Part model, mm, in its own coordinate system. Face numbers are marked on the shaded views. A direction names the side the tool comes from. Round coordinates to 2 decimals unless told otherwise and drop trailing zeros. Loops run counter-clockwise (first coordinate to the right, second up) from the corner with the lowest first, then second, coordinate; pieces in that order, holes last. Notation, with made-up numbers: (52.25, -9.75) -> (100.25, -9.75) arc R30 ccw to (100.25, 23.25) -> close; hole circle Ø3 at (19.25, 59.5). An arc over 180 degrees is marked (long way). Use a Markdown table: item, result. Add a question column.
Item 1: Cut at C-C, the plane y = 24. List the corners of the cut face in (x, z).
Item 2: Cut at B-B, the plane z = 16. List the corners of the cut face in (x, y).
Item 3: Flat gauge pins, fed straight in: pin 1 (1.6 mm diameter, centred on x = -27.5, z = 7.5, fed in from +Y); pin 2 (3.5 mm diameter, centred on x = -28.5, y = -2.5, fed in from +Z); pin 3 (3.5 mm diameter, centred on x = -28, z = 2.5, fed in from -Y). Where does each tip first touch, or does it go through?
Item 4: Probe line 1 (Y direction, x = 44, z = 6.75); line 2 (X direction, y = 17.5, z = 12.5); line 3 (Y direction, x = -3.5, z = 5.75). List the from-to ranges inside material, lowest first. Write a range as [from, to].
Item 5: Cut at A-A, the plane x = 26. List the corners of the cut face in (y, z), plus the area to 3 significant figures.
Item 6: Which spindle directions (+Z, -Z, +X, -X, +Y, -Y) get a long thin tool onto all of the face, cutting with end or side? Do the marked faces 1 and 2. Say none if no direction does.
Item 7: Cut at D-D, the plane y = 0. List the corners of the cut face in (x, z), plus the area to 3 significant figures.
Item 8: Two-plate mould, pull along X, no slides. Class the marked faces 3, 4, 5 and 6: pulls with the +X half, pulls with the -X half, needs draft (parallel to the pull), parting line crosses it, or undercut.
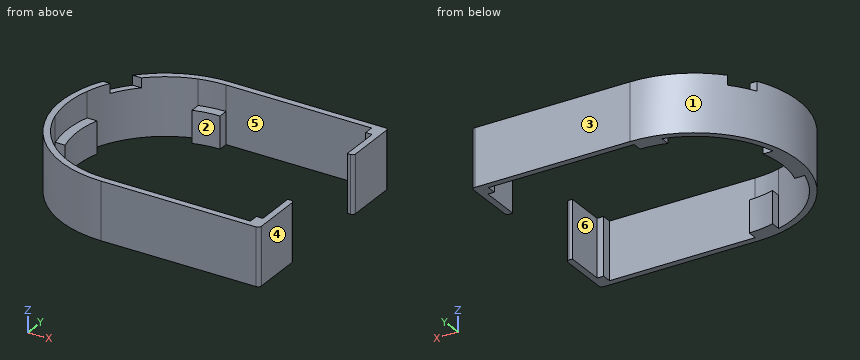
```python
from build123d import *

# Parameters (mm, degrees)
F1_DEPTH = 18
F2_R     = 1
F3_DEPTH = 10
F5_DEPTH = 3


with BuildPart() as f1:
    # F0 (on Top) → F1 (new body)
    with BuildSketch(Plane.XY):
        with BuildLine():
            Line((49.5, -32.5), (49.5, -15))
            Line((49.5, -15), (47.5, -15))
            Line((47.5, -15), (47.5, -27.5))
            Line((47.5, -27.5), (45.5, -27.5))
            Line((45.5, -27.5), (45.5, -30.5))
            Line((45.5, -30.5), (0, -30.5))
            ThreePointArc((0, -30.5), (-4.0354787933, -30.2318525881), (-8, -29.4321253055))
            ThreePointArc((-8, -29.4321253055), (-21.5667568262, -21.5667568262), (-29.4321253055, -8))
            ThreePointArc((-29.4321253055, -8), (-30.5, 0), (-29.4321253055, 8))
            ThreePointArc((-29.4321253055, 8), (-21.5667568262, 21.5667568262), (-8, 29.4321253055))
            ThreePointArc((-8, 29.4321253055), (-4.0354787933, 30.2318525881), (0, 30.5))
            Line((0, 30.5), (45.5, 30.5))
            Line((45.5, 30.5), (45.5, 27.5))
            Line((45.5, 27.5), (47.5, 27.5))
            Line((47.5, 27.5), (47.5, 15))
            Line((47.5, 15), (49.5, 15))
            Line((49.5, 15), (49.5, 32.5))
            Line((49.5, 32.5), (0, 32.5))
            ThreePointArc((0, 32.5), (-32.5, 0), (0, -32.5))
            Line((0, -32.5), (49.5, -32.5))
        make_face()
    extrude(amount=F1_DEPTH)

    # F2
    f2_edges = [f1.edges().sort_by_distance(p)[0] for p in [
        (49.5, 15, 9),
        (49.5, -15, 9),
        (49.5, 32.5, 9),
        (49.5, -32.5, 9),
    ]]
    fillet(f2_edges, radius=F2_R)

    # F0 (on Top) → F3 (join)
    with BuildSketch(Plane.XY):
        with BuildLine():
            ThreePointArc((0, 30.5), (-4.0354787933, 30.2318525881), (-8, 29.4321253055))
            Line((-8, 29.4321253055), (-8, 26.3106442338))
            ThreePointArc((-8, 26.3106442338), (-4.0439636231, 27.2010359769), (0, 27.5))
            Line((0, 27.5), (0, 30.5))
        make_face()
        with BuildLine():
            ThreePointArc((-29.4321253055, 8), (-30.5, 0), (-29.4321253055, -8))
            Line((-29.4321253055, -8), (-26.3106442338, -8))
            ThreePointArc((-26.3106442338, -8), (-27.5, 0), (-26.3106442338, 8))
            Line((-26.3106442338, 8), (-29.4321253055, 8))
        make_face()
        with BuildLine():
            ThreePointArc((-8, -29.4321253055), (-4.0354787933, -30.2318525881), (0, -30.5))
            Line((0, -30.5), (0, -27.5))
            ThreePointArc((0, -27.5), (-4.0439636231, -27.2010359769), (-8, -26.3106442338))
            Line((-8, -26.3106442338), (-8, -29.4321253055))
        make_face()
    extrude(amount=F3_DEPTH)

    # F4 (on face) → F5 (cut)
    with BuildSketch(Plane.XY.offset(18)):
        with BuildLine():
            Line((-28.8314064867, 15), (-26.5565434498, 15))
            ThreePointArc((-26.5565434498, 15), (-24.0961320452, 18.698299935), (-21.1246301743, 22))
            Line((-21.1246301743, 22), (-23.9217474278, 22))
            ThreePointArc((-23.9217474278, 22), (-26.6077772837, 18.6621592539), (-28.8314064867, 15))
        make_face()
    extrude(amount=-F5_DEPTH, mode=Mode.SUBTRACT)


solid = f1.part
```
A:
| question | item | result |
|---|---|---|
| 1 | outline | (-21.91, 0) -> (-18.82, 0) -> (-18.82, 18) -> (-21.91, 18) -> close; (47.5, 0) -> (49.5, 0) -> (49.5, 18) -> (47.5, 18) -> close |
| 2 | outline | (-28.83, 15) arc R32.5 ccw to (0, -32.5) -> (48.5, -32.5) arc R1 ccw to (49.5, -31.5) -> (49.5, -16) arc R1 ccw to (48.5, -15) -> (47.5, -15) -> (47.5, -27.5) -> (45.5, -27.5) -> (45.5, -30.5) -> (0, -30.5) arc R30.5 cw to (-26.56, 15) -> close; (-23.92, 22) -> (-21.12, 22) arc R30.5 cw to (0, 30.5) -> (45.5, 30.5) -> (45.5, 27.5) -> (47.5, 27.5) -> (47.5, 15) -> (48.5, 15) arc R1 ccw to (49.5, 16) -> (49.5, 31.5) arc R1 ccw to (48.5, 32.5) -> (0, 32.5) arc R32.5 ccw to start |
| 3 | pin 1 | stops at y = 18.53 |
| 3 | pin 2 | stops at z = 10 |
| 3 | pin 3 | stops at y = -19.16 |
| 4 | line 1 | y = [-32.5, -30.5], [30.5, 32.5] |
| 4 | line 2 | x = [-27.39, -24.98], [47.5, 49.5] |
| 4 | line 3 | y = [-32.31, -27.28], [27.28, 32.31] |
| 5 | outline | (-32.5, 0) -> (-30.5, 0) -> (-30.5, 18) -> (-32.5, 18) -> close; (30.5, 0) -> (32.5, 0) -> (32.5, 18) -> (30.5, 18) -> close |
| 5 | area | 72.0 mm^2 |
| 6 | face 1 | +Z, -Z, -X |
| 6 | face 2 | +Z, -Z |
| 7 | outline | (-32.5, 0) -> (-27.5, 0) -> (-27.5, 10) -> (-30.5, 10) -> (-30.5, 18) -> (-32.5, 18) -> close |
| 7 | area | 66.0 mm^2 |
| 8 | face 3 | needs draft |
| 8 | face 4 | pulls with the +X half |
| 8 | face 5 | undercut |
| 8 | face 6 | undercut |
